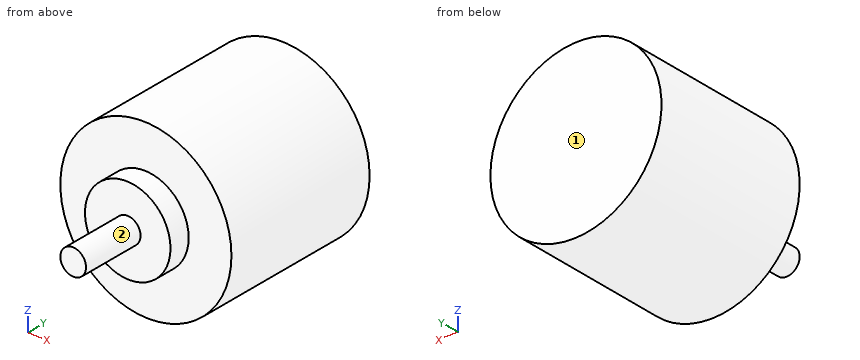
```python
from build123d import *

# Parameters (mm, degrees)
ESBO_O11_R               = 20
RESSALTO_EXTRUS_O3_DEPTH = 38
ESBO_O12_R               = 10
RESSALTO_EXTRUS_O4_DEPTH = 5
ESBO_O13_R               = 3
RESSALTO_EXTRUS_O5_DEPTH = 15


with BuildPart() as part:
    # Esboço11 → Ressalto-extrusão3 (new body)
    with BuildSketch(Plane.XZ):
        Circle(ESBO_O11_R)
    extrude(amount=RESSALTO_EXTRUS_O3_DEPTH)

    # Esboço12 → Ressalto-extrusão4 (add)
    with BuildSketch(Plane.XZ.offset(38)):
        Circle(ESBO_O12_R)
    extrude(amount=RESSALTO_EXTRUS_O4_DEPTH)

    # Esboço13 → Ressalto-extrusão5 (add)
    with BuildSketch(Plane.XZ.offset(43)):
        Circle(ESBO_O13_R)
    extrude(amount=RESSALTO_EXTRUS_O5_DEPTH)


solid = part.part
```
Geometry check sheet. Reference: the model listing, model coordinates, mm. Face numbers are marked on the shaded views. A direction names the side the tool comes from. Coordinates: 2 decimals unless noted, no trailing zeros. Order: outer loops, then holes, each group sorted by start corner. A loop starts at its lowest first (then second) coordinate and runs counter-clockwise, first axis right, second up.
Q1. Sectioned sample at C-C on y = -21.5. Record the cut outline in (x, z), and give its area (3 significant figures).
Reply:
outline: circle Ø40 at (0, 0)
area: 1,260 mm2
Q2. Thickness scan on probe 1 along Y at (x, z) = (12.5, 8); probe 2 along Y at (x, z) = (-6, 5); probe 3 along Z at (x, y) = (0, -6.5). Record the ranges inside material, lowest first.
Reply:
probe 1: y = -38 to 0
probe 2: y = -43 to 0
probe 3: z = -20 to 20
Q3. Sectioned sample at D-D on x = -5. Record the cut outline in (y, z), and give its area (3 significant figures).
Reply:
outline: (-43, -8.66) - (-38, -8.66) - (-38, -19.36) - (0, -19.36) - (0, 19.36) - (-38, 19.36) - (-38, 8.66) - (-43, 8.66) - close
area: 1,560 mm2
Q4. Tool access check on the marked faces 1 and 2. Record the directions out of +Z, -Z, +X, -X, +Y, -Y that give a thin tool (end or side, any length) a straight path to the whole face; none if there is none.
Reply:
face 1: +Z, -Z, +X, -X, +Y
face 2: -Y
Q5. Sectioned sample at A-A on x = 0. Record the cut outline in (y, z), and give its area (3 significant figures).
Reply:
outline: (-58, -3) - (-43, -3) - (-43, -10) - (-38, -10) - (-38, -20) - (0, -20) - (0, 20) - (-38, 20) - (-38, 10) - (-43, 10) - (-43, 3) - (-58, 3) - close
area: 1,710 mm2
Q6. Sectioned sample at B-B on z = 0. Record the cut outline in (x, y).
Reply:
outline: (-20, -38) - (-10, -38) - (-10, -43) - (-3, -43) - (-3, -58) - (3, -58) - (3, -43) - (10, -43) - (10, -38) - (20, -38) - (20, 0) - (-20, 0) - close
Q7. Depth check by flat-ended pin: pin 1 Ø1.5 at (y, z) = (-32, 10) entering from +X; pin 2 Ø6 at (y, z) = (-17, -10.5) entering from -X; pin 3 Ø5 at (x, y) = (-12, -20) entering from +Z. Enter the tip coordinate at first touch or a pass-through.
Reply:
pin 1: stops at x = 17.73
pin 2: stops at x = -18.54
pin 3: stops at z = 17.6
